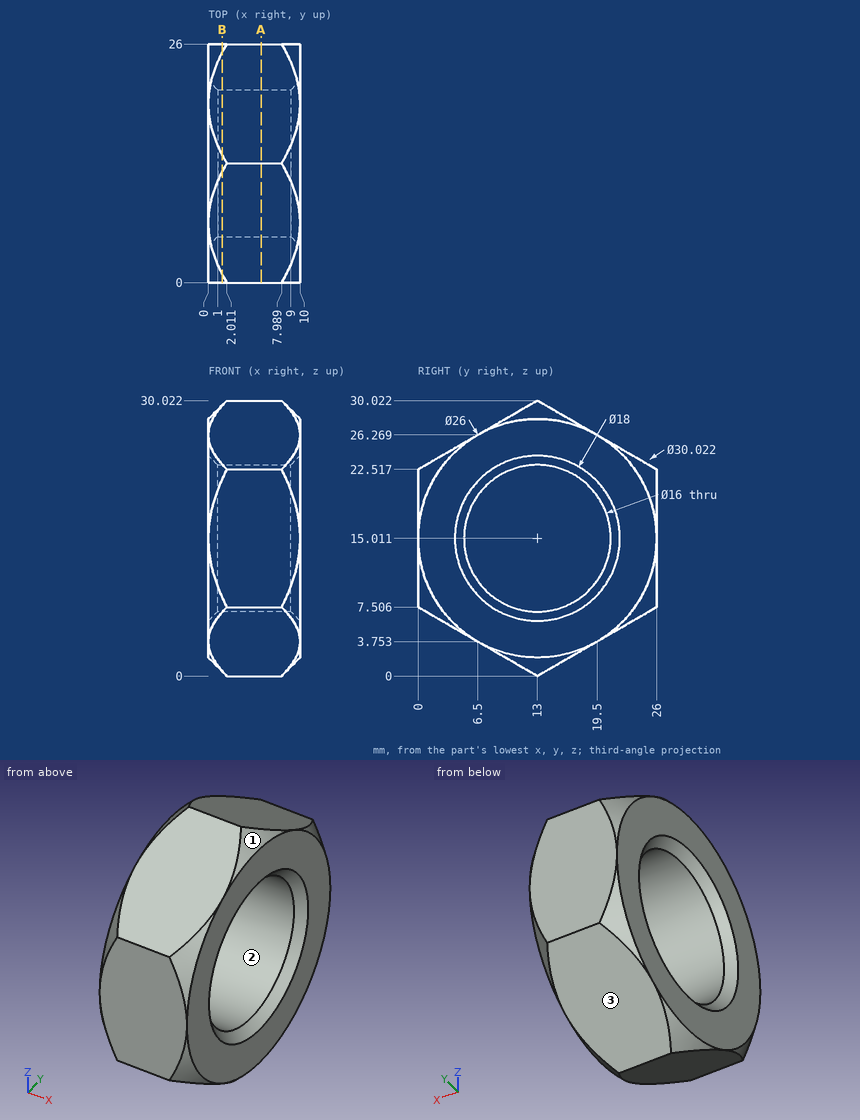
For this review, use the dimensioned drawing (mm, ordinates from the lowest corner) and the shaded views. Give positions to 0.01 mm unless a question says otherwise; leave off trailing zeros. Order: outer loops, then holes, each group sorted by start corner. A loop starts at its lowest first (then second) coordinate and runs counter-clockwise, first axis right, second up.
1) Take a section at A-A (x = 5.75). Give the boundary of the cut face in (y, z) (1 decimal), then the cut area to 3 significant figures.
2) Wall thickness on line 1 (Y direction, x = 5.5, z = 15); line 2 (Y direction, x = 5.5, z = 21) (1 decimal); line 3 (Z direction, x = 6.75, y = 15.75) (1 decimal): over which ranges is each line inside the solid? List them lowest first.
3) Take a section at B-B (x = 1.5). Give the boundary of the cut face in (y, z).
4) Insertion check: pin 1 (1 mm diameter, centred on x = 9, y = 16, fed in from -Z); pin 2 (2 mm diameter, centred on x = 2.5, y = 22.5, fed in from -Z); pin 3 (4 mm diameter, centred on x = 2, y = 15.5, fed in from -Z). Each pin has a flat end and moves straight along its axis. Give the tip position at first contact, or say it passes through.
5) The part is to be moulded in two halves that separate along Z. For the marked faces 1, 2 and 3, say which applies: released by +Z, released by -Z, zero draft, split by the parting line, or undercut.
Derived:
1. outline: (0, 7.5) - (13, 0) - (26, 7.5) - (26, 22.5) - (13, 30) - (0, 22.5) - close; hole circle Ø16 at (13, 15)
1. area: 384 mm2
2. line 1: y = 0 to 5, 21 to 26
2. line 2: y = 0 to 7.7, 18.3 to 26
2. line 3: z = 1.6 to 7.5, 22.5 to 28.4
3. outline: (0, 8.59) arc R14.5 ccw to (0.94, 6.96) - (12.06, 0.54) arc R14.5 ccw to (13.94, 0.54) - (25.06, 6.96) arc R14.5 ccw to (26, 8.59) - (26, 21.43) arc R14.5 ccw to (25.06, 23.06) - (13.94, 29.48) arc R14.5 ccw to (12.06, 29.48) - (0.94, 23.06) arc R14.5 ccw to (0, 21.43) - close; hole circle Ø16 at (13, 15.01)
4. pin 1: stops at z = 1.44
4. pin 2: stops at z = 4.91
4. pin 3: stops at z = 0.29
5. face 1: released by +Z
5. face 2: undercut
5. face 3: released by -Z
